```python
from build123d import *

# Parameters (mm, degrees)
F0_R     = 10
F0_R_2   = 15
F1_DEPTH = 30


with BuildPart() as f1:
    # F0 (on Front) → F1 (new body)
    with BuildSketch(Plane.XZ):
        with BuildLine():
            ThreePointArc((-81.915204, 32.357644), (-44.077123, 21.298231), (-18.151285, -8.398265))
            ThreePointArc((-18.151285, -8.398265), (-0.902184, -19.979641), (17.320508, -10))
            Line((17.320508, -10), (67.320508, 76.60254))
            ThreePointArc((67.320508, 76.60254), (69.442127, 91.293348), (60.854969, 103.400446))
            ThreePointArc((60.854969, 103.400446), (-27.111474, 120.420007), (-102.346878, 71.764126))
            ThreePointArc((-102.346878, 71.764126), (-104.109371, 45.850299), (-81.915204, 32.357644))
        make_face()
        Circle(F0_R, mode=Mode.SUBTRACT)
        with Locations((-81.915204, 57.357644)):
            Circle(F0_R_2, mode=Mode.SUBTRACT)
        with BuildLine():
            ThreePointArc((-69.260057, 78.91796), (-20.13831, 103.050708), (34.45473, 99.186045))
            ThreePointArc((34.45473, 99.186045), (30.879167, 80.737922), (44.183374, 67.467053))
            Line((44.183374, 67.467053), (13.663505, 14.605089))
            ThreePointArc((13.663505, 14.605089), (-2.403826, 19.855015), (-16.754099, 10.922461))
            ThreePointArc((-16.754099, 10.922461), (-35.823115, 31.52567), (-61.436403, 43.018233))
            ThreePointArc((-61.436403, 43.018233), (-57.488534, 62.680966), (-69.260057, 78.91796))
        make_face(mode=Mode.SUBTRACT)
        with Locations((50, 86.60254)):
            Circle(F0_R, mode=Mode.SUBTRACT)
    extrude(amount=F1_DEPTH)


solid = f1.part
```
CAD build for the part. Positions are in the model's coordinates, mm. A direction names the side the tool comes from. Round coordinates to 2 decimals unless told otherwise and drop trailing zeros. Loops run counter-clockwise (first coordinate to the right, second up) from the corner with the lowest first, then second, coordinate; pieces in that order, holes last. Notation, with made-up numbers: M -22.75,61 L -13.75,61 A16 cw -13.75,80 Z; hole C 18,12 d5. An arc over 180 degrees is marked long. Return JSON: item names as keys, results as strings. Group by question number.
(1) Tool access for faces 4 (the flat face through (29.14, -14.79, 41.41)), 5 (the flat face through (41.971, -14.79, 32.695)): list every direction of +Z, -Z, +X, -X, +Y, -Y with a clear straight run to the whole face (end or side of a thin tool).
(2) Wall check: probe 1 along X at (y, z) = (-27, 43.5); probe 2 along Z at (x, y) = (0, -20); probe 3 along X at (y, z) = (-21.25, 66). Give the ranges that are in metal, low to high. Write a range as [from, to].
(3) Drop flat-ended pins along their axis: P1, Ø2, axis at x = 5, y = -25, coming from the +Z side; P2, Ø8, axis at y = -12.5, z = 89.5, coming from the -X side; P3, Ø6, axis at y = -6, z = 72, coming from the +X side; P4, Ø8, axis at x = 28, z = -2.5, coming from the +Y side. Give the stop position or say it passes through.
(4) Saw through at A-A, the plane z = 55. List the corners of the cut face in (x, y).
(5) Saw through at C-C, the plane x = 0. List the corners of the cut face in (y, z).
(6) Mould opens along Z. For faces 1 (the cylindrical face through (-25.848, -14.79, 120.658)), 2 (the cylindrical face through (-44.55, -14.79, 21.6)), 3 (the cylindrical face through (-2.161, -14.79, 19.883)) say: +Z half, -Z half, draft (parallel to the pull), parting line (faces both ways), or undercut.
(7) Saw through at D-D, the plane z = 34.5. List the corners of the cut face in (x, y).
(8) Saw through at B-B, the plane x = 50. List the corners of the cut face in (y, z), and give its area (3 significant figures).
Answer list:
{
 "1": {"face 4": "+Y, -Y", "face 5": "-Z, +X, +Y, -Y"},
 "2": {"probe 1": "[-102.72, -87.66], [-76.17, -61.11], [30.35, 48.21]", "probe 2": "[-20, -10], [10, 20], [105, 122.54]", "probe 3": "[-105.37, -94.18], [-69.66, -58.46], [43.34, 61.2]"},
 "3": {"P1": "z = 122.33", "P2": "x = -91.05", "P3": "x = 66.4", "P4": "through"},
 "4": {"outline": "M -106.8,-30 L -96.73,-30 L -96.73,0 L -106.8,0 Z; M -67.1,-30 L -57.03,-30 L -57.03,0 L -67.1,0 Z; M 36.99,-30 L 54.85,-30 L 54.85,0 L 36.99,0 Z"},
 "5": {"outline": "M -30,-20 L 0,-20 L 0,-10 L -30,-10 Z; M -30,10 L 0,10 L 0,20 L -30,20 Z; M -30,105 L 0,105 L 0,122.54 L -30,122.54 Z"},
 "6": {"face 1": "+Z half", "face 2": "-Z half", "face 3": "undercut"},
 "7": {"outline": "M -92.04,-30 L -40.32,-30 L -40.32,0 L -92.04,0 Z; M 25.15,-30 L 43.01,-30 L 43.01,0 L 25.15,0 Z"},
 "8": {"outline": "M -30,46.6 L 0,46.6 L 0,76.6 L -30,76.6 Z; M -30,96.6 L 0,96.6 L 0,109.64 L -30,109.64 Z", "area": "1,290 mm2"}
}
